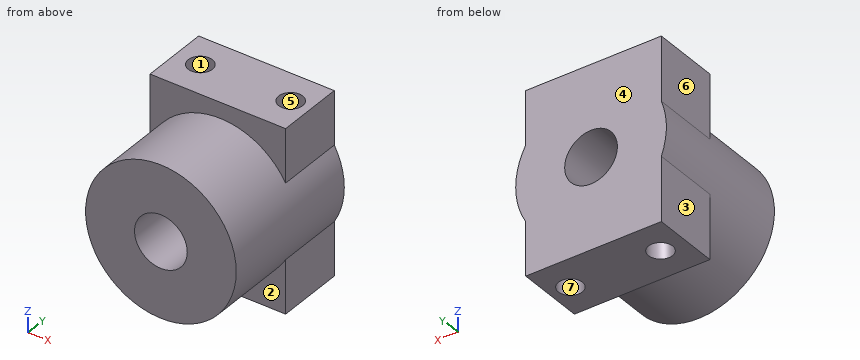
from build123d import *

# Parameters (mm, degrees)
F0_R     = 10
F0_R_2   = 3.5
F1_DEPTH = 20
F2_W     = 18
F2_H     = 8.5
F3_DEPTH = 9
F4_R     = 1.6
F5_DEPTH = 4
F6_R     = 1.6
F7_DEPTH = 4


with BuildPart() as f1:
    # F0 (on Front) → F1 (new body)
    with BuildSketch(Plane.XZ):
        Circle(F0_R)
        Circle(F0_R_2, mode=Mode.SUBTRACT)
    extrude(amount=F1_DEPTH)

    # F2 (on Front) → F3 (join)
    with BuildSketch(Plane.XZ):
        with Locations((-0.332717, 7.839034)):
            Rectangle(F2_W, F2_H)
        with Locations((-0.332717, -7.839034)):
            Rectangle(F2_W, F2_H)
    extrude(amount=F3_DEPTH)

    # F4 (on face) → F5 (cut)
    with BuildSketch(Plane.XY.offset(12.089034)):
        with Locations((-5.996018, -4.33991)):
            Circle(F4_R)
        with Locations((5.996018, -4.33991)):
            Circle(F4_R)
    extrude(amount=-F5_DEPTH, mode=Mode.SUBTRACT)

    # F6 (on face) → F7 (cut)
    with BuildSketch(Plane(origin=(0, 0, -12.089034), x_dir=(1, 0, 0), z_dir=(0, 0, -1))):
        with Locations((5.982172, 4.523708)):
            Circle(F6_R)
        with Locations((-5.982172, 4.523708)):
            Circle(F6_R)
    extrude(amount=-F7_DEPTH, mode=Mode.SUBTRACT)


solid = f1.part
Verification items for the finished model (mm, model axes). Face numbers are marked on the shaded views. A direction names the side the tool comes from. Coordinates: 2 decimals unless noted, no trailing zeros. Loops run counter-clockwise (first coordinate to the right, second up) from the corner with the lowest first, then second, coordinate; pieces in that order, holes last. Notation, with made-up numbers: M -30.5,23.5 L -25.5,23.5 A31 ccw -25.5,59.5 Z; hole C 76,4 d5. An arc over 180 degrees is marked long. One line per item, written item: value.
1. Section check A-A on x = 0. Record the cut outline in (y, z).
Answers follow:
outline: M -20,-10 L -9,-10 L -9,-12.09 L 0,-12.09 L 0,-3.5 L -20,-3.5 Z; M -20,3.5 L 0,3.5 L 0,12.09 L -9,12.09 L -9,10 L -20,10 Z
2. Set-up check for the marked faces 5, 6 and 7: record each of +Z, -Z, +X, -X, +Y, -Y from which the full face is reachable in a straight line by a thin tool's end or side.
Answers follow:
face 5: +Z
face 6: +Z, -X, +Y, -Y
face 7: -Z
3. Section check D-D on z = 6. Record the cut outline in (x, y).
Answers follow:
outline: M -9.33,-9 L -8,-9 L -8,-20 L 8,-20 L 8,-9 L 8.67,-9 L 8.67,0 L -9.33,0 Z
4. Material ranges on line 1 along Z through (x, y) = (0, -11.5); line 2 along Z through (x, y) = (-1.75, -10.5); line 3 along Y through (x, z) = (-9, 10), recorded low to high. Write a range as from..to.
Answers follow:
line 1: -10..-3.5, 3.5..10
line 2: -9.85..-3.03, 3.03..9.85
line 3: -9..0
5. Gauge pin test, flat ends, axial feed: P1, Ø3.5, axis at y = -2.5, z = 10, coming from the +X side; P2, Ø2.5, axis at y = -5, z = -6, coming from the -X side; P3, Ø2.5, axis at x = -5.98, y = -4.52, coming from the +Z side. Record the tip position at first contact, or that the pin passes through.
Answers follow:
P1: x = 8.67
P2: x = -9.33
P3: z = 8.09
6. Section check B-B on z = 0. Record the cut outline in (x, y), plus the area to 3 significant figures.
Answers follow:
outline: M -10,-20 L -3.5,-20 L -3.5,0 L -10,0 Z; M 3.5,-20 L 10,-20 L 10,0 L 3.5,0 Z
area: 260 mm^2
7. Mould release check, pull along Y, two halves, no side actions. Record for the marked faces 1, 2, 3 and 4: pulls with the +Y half, pulls with the -Y half, needs draft (parallel to the pull), parting line crosses it, or undercut.
Answers follow:
face 1: undercut
face 2: pulls with the -Y half
face 3: needs draft
face 4: pulls with the +Y half
8. Section check C-C on y = -8. Record the cut outline in (x, z), plus the area to 3 significant figures.
Answers follow:
outline: M -9.33,-12.09 L 8.67,-12.09 L 8.67,-4.99 A10 ccw 8.67,4.99 L 8.67,12.09 L -9.33,12.09 L -9.33,3.59 A10 ccw -9.33,-3.59 Z; hole C 0,0 d7
area: 409 mm^2
